The model under review builds one solid part; all positions refer to its coordinate system, in mm. Face numbers are marked on the shaded views. A direction names the side the tool comes from. Coordinates: 2 decimals unless noted, no trailing zeros. Loops run counter-clockwise (first coordinate to the right, second up) from the corner with the lowest first, then second, coordinate; pieces in that order, holes last. Notation, with made-up numbers: M -15.75,-18 L 41.25,-18 A15 ccw 41.25,11 Z; hole C 52.5,-13 d3. An arc over 180 degrees is marked long. Return JSON: item names as keys, results as strings.
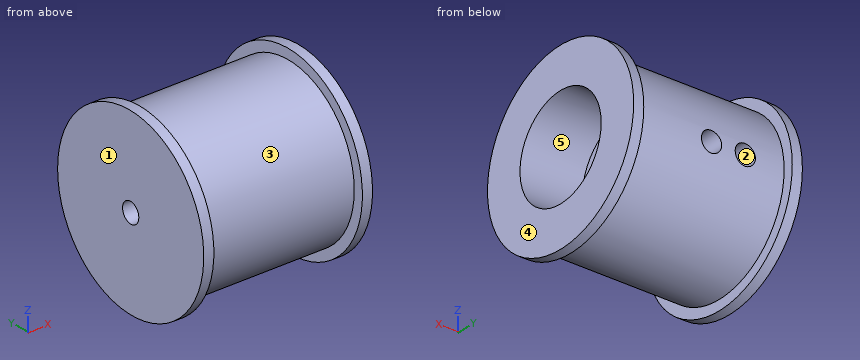
Autodesk Inventor part; units mm, degrees
ref_plane "Pracovní rovina1" through (12.5, 12, 0) normal (0, 1, 0) x (-1, 0, 0)
ref_plane "YZ Plane" through (0, 0, 0) normal (1, 0, 0) x (0, 1, 0)
ref_plane "XY Plane" through (0, 0, 0) normal (0, 0, 1) x (1, 0, 0)
sketch "Náčrt1" plane through (0, 0, 0) normal (0, 0, 1) x (1, 0, 0)
  line L0 (0, 0) -> (25, 0)
  line L1 (0, 0) -> (0, 13.5)
  line L2 (0, 13.5) -> (1.5, 13.5)
  line L3 (1.5, 13.5) -> (1.5, 12)
  line L4 (1.5, 12) -> (23.5, 12)
  line L5 (23.5, 12) -> (23.5, 13.5)
  line L6 (23.5, 13.5) -> (25, 13.5)
  line L7 (25, 13.5) -> (25, 7.5)
  line L8 (25, 7.5) -> (15.75, 7.5)
  line L9 (48.5, 7.4) -> (48.5, -7.4) construction
  line L10 (6.5, 1.5) -> (6.5, -1.5) construction
  line L11 (15.75, 7.4) -> (15.75, -7.4) construction
  line L12 (6.5, 1.5) -> (15.75, 1.5) construction
  line L13 (6.5, -1.5) -> (15.75, -1.5) construction
  line L14 (15.75, 7.5) -> (15.75, 0)
  line L15 (13.75, 12) -> (13.75, 1.5) construction
  line L16 (10.75, 1.5) -> (10.75, 12) construction
  line L17 (8.75, 12) -> (8.75, 1.5) construction
  line L18 (5.75, 1.5) -> (5.75, 12) construction
  line L19 (15.75, 1.5) -> (0, 1.5)
  line L20 (5.75, 12) -> (7.25, 12) construction
  line L21 (7.25, 12) -> (8.75, 12) construction
  line L22 (12.25, 12) -> (10.75, 12) construction
  line L23 (12.25, 12) -> (13.75, 12) construction
  point P0 (6.5, 0)
  point P1 (24.25, 13.5)
  point P2 (15.75, 1.5)
  dimension "d1" = 15
  dimension "d2" = 48.5
  dimension "d3" = 42
  dimension "d4" = 3
  dimension "d5" = 9.25
  dimension "d6" = 14.8
  dimension "d7" = 27
  dimension "d8" = 25
  dimension "d9" = 1.5
  dimension "d10" = 1.5
  dimension "d11" = 3
  dimension "d12" = 2
  dimension "d13" = 3
  dimension "d14" = 2
revolve "Rotace1" add sketch "Náčrt1" angle 360 about axis through (0, 0, 0) along (1, 0, 0) contours L1 L2 L3 L4 L5 L6 L7 L8 L14 L19
ref_plane "Pracovní rovina1" through (12.5, 12, 0) normal (0, 1, 0) x (-1, 0, 0)
sketch "Náčrt2" plane through (12.5, 12, 0) normal (0, 1, 0) x (-1, 0, 0)
  point P0 (12.5, 0)
  point P1 (5.25, 0)
  point P2 (0.25, 0)
hole "Díra1" at (7.25, 12, 0) at (12.25, 12, 0) direction (0, -1, 0) diameter 3 depth 12
thread "Závit1"
thread "Závit2"
properties part number "wheelGen2" material "Mosaz, měkká žlutá"
1. The part is to be moulded in two halves that separate along Y. For the marked faces 3, 4 and 5, say which applies: released by +Y, released by -Y, zero draft, split by the parting line, or undercut.
Check values:
{"face 3": "split by the parting line", "face 4": "zero draft", "face 5": "undercut"}
2. To check wall thickness, follow line 1 (X direction, y = 9.75, z = 0); line 2 (X direction, y = -12.5, z = 1.5); line 3 (Z direction, x = 21, y = 0). State the ranges of each line that lie inside material, in increasing order.
Check values:
{"line 1": "0 to 5.75, 8.75 to 10.75, 13.75 to 25", "line 2": "0 to 1.5, 23.5 to 25", "line 3": "-12 to -7.5, 7.5 to 12"}
3. Add section D-D on y = 4.25. Give the boundary of the cut face in (x, z), plus the area to 3 significant figures.
Check values:
{"outline": "M 0,-12.81 L 1.5,-12.81 L 1.5,-11.22 L 23.5,-11.22 L 23.5,-12.81 L 25,-12.81 L 25,-6.18 L 15.75,-6.18 L 15.75,6.18 L 25,6.18 L 25,12.81 L 23.5,12.81 L 23.5,11.22 L 1.5,11.22 L 1.5,12.81 L 0,12.81 Z; hole C 7.25,0 d3; hole C 12.25,0 d3", "area": "442 mm²"}
4. Machinability: for the marked faces 1 and 2, which of the approach directions +Z, -Z, +X, -X, +Y, -Y give a long, thin tool a straight path to every point of the face, cutting with its end or side? Answer none if there is none.
Check values:
{"face 1": "+Z, -Z, -X, +Y, -Y", "face 2": "+Y"}
5. Add section C-C on y = -4.25. Give the boundary of the cut face in (x, z), plus the area to 3 significant figures.
Check values:
{"outline": "M 0,-12.81 L 1.5,-12.81 L 1.5,-11.22 L 23.5,-11.22 L 23.5,-12.81 L 25,-12.81 L 25,-6.18 L 15.75,-6.18 L 15.75,6.18 L 25,6.18 L 25,12.81 L 23.5,12.81 L 23.5,11.22 L 1.5,11.22 L 1.5,12.81 L 0,12.81 Z", "area": "456 mm²"}
6. Add section B-B on x = 10.25. Give the boundary of the cut face in (y, z), plus the area to 3 significant figures.
Check values:
{"outline": "C 0,0 d24; hole C 0,0 d3", "area": "445 mm²"}
7. Insertion check: pin 1 Ø3.5 at (x, z) = (7.25, 0) entering from +Y; pin 2 Ø8 at (x, y) = (6, 10) entering from +Z; pin 3 Ø3.5 at (y, z) = (0, 0) entering from +X. Each pin has a flat end and moves straight along its axis. Give the tip position at first contact, or say it passes through.
Check values:
{"pin 1": "y = 12", "pin 2": "z = 10.39", "pin 3": "x = 15.75"}
8. Add section A-A on z = 0. Give the boundary of the cut face in (x, y).
Check values:
{"outline": "M 0,-13.5 L 1.5,-13.5 L 1.5,-12 L 23.5,-12 L 23.5,-13.5 L 25,-13.5 L 25,-7.5 L 15.75,-7.5 L 15.75,-1.5 L 0,-1.5 Z; M 0,1.5 L 5.75,1.5 L 5.75,12 L 1.5,12 L 1.5,13.5 L 0,13.5 Z; M 8.75,1.5 L 10.75,1.5 L 10.75,12 L 8.75,12 Z; M 13.75,1.5 L 15.75,1.5 L 15.75,7.5 L 25,7.5 L 25,13.5 L 23.5,13.5 L 23.5,12 L 13.75,12 Z"}
